from build123d import *

# Parameters (mm, degrees)
SKETCH1_R               = 150
BOSS_EXTRUDE1_DEPTH     = 50
SHELL2_T                = -5
FILLET1_R               = 10
SKETCH4_R               = 3
SKETCH4_R_2             = 1.25
CUT_EXTRUDE2_DEPTH      = 218.944947177
CUT_EXTRUDE2_DEPTH_BACK = 218.944947177
SKETCH5_W               = 60
SKETCH5_H               = 3
CUT_EXTRUDE3_DEPTH      = 218.944947177
CUT_EXTRUDE3_DEPTH_BACK = 218.944947177


with BuildPart() as part:
    # Sketch1 → Boss-Extrude1 (new body)
    with BuildSketch(Plane(origin=(0, 0, 0), x_dir=(1, 0, 0), z_dir=(0, 1, 0))):
        with Locations(Location((0, 0, 0), (0, 0, 270))):
            Circle(SKETCH1_R)
    extrude(amount=BOSS_EXTRUDE1_DEPTH)

    # Shell2
    shell2_openings = [part.faces().sort_by_distance(p)[0] for p in [
        (0, 0, 0),
    ]]
    offset(amount=SHELL2_T, openings=shell2_openings, kind=Kind.INTERSECTION)

    # Fillet1
    fillet1_edges = [part.edges().sort_by_distance(p)[0] for p in [
        (0, 50, -150),
        (0, 45, -145),
    ]]
    fillet(fillet1_edges, radius=FILLET1_R)

    # Sketch4 → Cut-Extrude2 (cut, two sides)
    with BuildSketch(Plane(origin=(0, 50, 0), x_dir=(1, 0, 0), z_dir=(0, 1, 0))) as cut_extrude2_sk:
        with Locations(Location((-22, 31, 0), (0, 0, 270))):
            Circle(SKETCH4_R)
        with Locations(Location((35, 25, 0), (0, 0, 270))):
            Circle(SKETCH4_R)
        with Locations(Location((-22, -31, 0), (0, 0, 270))):
            Circle(SKETCH4_R)
        with Locations(Location((35, -25, 0), (0, 0, 270))):
            Circle(SKETCH4_R)
        with Locations(Location((0, -60, 0), (0, 0, 270))):
            Circle(SKETCH4_R_2)
        with Locations(Location((-15, -75, 0), (0, 0, 270))):
            Circle(SKETCH4_R_2)
        with Locations(Location((0, -90, 0), (0, 0, 270))):
            Circle(SKETCH4_R_2)
        with Locations(Location((15, -75, 0), (0, 0, 270))):
            Circle(SKETCH4_R_2)
    extrude(amount=CUT_EXTRUDE2_DEPTH, mode=Mode.SUBTRACT)
    extrude(cut_extrude2_sk.sketch, amount=-CUT_EXTRUDE2_DEPTH_BACK, mode=Mode.SUBTRACT)

    # Sketch5 → Cut-Extrude3 (cut, two sides)
    with BuildSketch(Plane(origin=(0, 0, 0), x_dir=(0, 0, -1), z_dir=(1, 0, 0))) as cut_extrude3_sk:
        with Locations((0, 15)):
            Rectangle(SKETCH5_W, SKETCH5_H)
        with Locations((0, 10.5)):
            Rectangle(SKETCH5_W, SKETCH5_H)
        with Locations((0, 19.5)):
            Rectangle(SKETCH5_W, SKETCH5_H)
    extrude(amount=CUT_EXTRUDE3_DEPTH, mode=Mode.SUBTRACT)
    extrude(cut_extrude3_sk.sketch, amount=-CUT_EXTRUDE3_DEPTH_BACK, mode=Mode.SUBTRACT)


solid = part.part
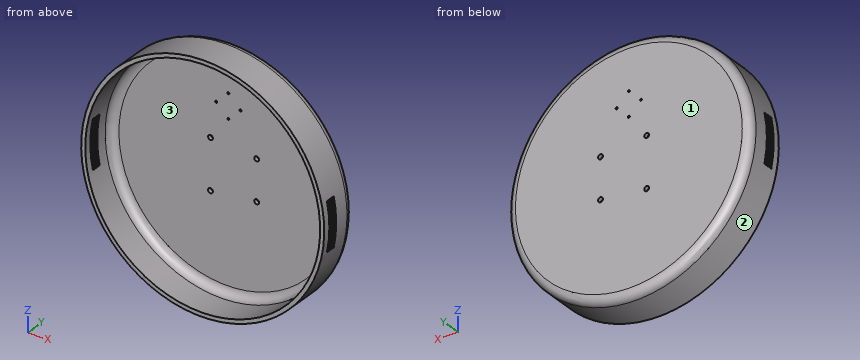
The listing builds one solid part. Answer for the finished solid, in the listing's coordinates (mm). Face numbers are marked on the shaded views. Coordinates: 2 decimals unless noted, no trailing zeros. Answer in a Markdown table with one row per item. Add a question column.
1. Determine the mould class of the marked faces 1, 2 and 3 for opening direction Z: +Z half, -Z half, draft (parallel to the pull), parting line (faces both ways), or undercut.
2. Flat-ended cylindrical pins translate along their axes: P1, Ø2, axis at y = 41.5, z = 101.5, coming from the +X side; P2, Ø12, axis at x = -116, y = 23, coming from the -Z side; P3, Ø2, axis at x = -15, z = 75, coming from the -Y side; P4, Ø2.5, axis at x = 144.5, z = 2.5, coming from the +Y side. Find the tip coordinate at first contact, or state that the pin passes through.
3. Consider line 1 (X direction, y = 46.6, z = 75); line 2 (X direction, y = 47.5, z = 75); line 3 (Z direction, x = -130.5, y = 3). Determine where each line is inside the solid, lowest interval first. Write a range as [from, to].
4. The part is cut by section A-A, the plane z = 0. Count the separate pieces of the cut face and the enclosed holes in it, then the cut area to 3 significant figures.
Answer below:
| question | item | result |
|---|---|---|
| 1 | face 1 | draft |
| 1 | face 2 | parting line |
| 1 | face 3 | undercut |
| 2 | P1 | x = 111.22 |
| 2 | P2 | z = -101.98 |
| 2 | P3 | through |
| 2 | P4 | y = 49.45 |
| 3 | line 1 | [-127.02, -16.25], [-13.75, 13.75], [16.25, 127.02] |
| 3 | line 2 | [-125.98, -16.25], [-13.75, 13.75], [16.25, 125.98] |
| 3 | line 3 | [-73.96, -63.2], [63.2, 73.96] |
| 4 | separate pieces | 7 |
| 4 | enclosed holes | 0 |
| 4 | area | 1,860 mm2 |
